Autodesk Fusion 360 part; units mm, degrees
sketch "Sketch1" plane through (0, 0, 0) normal (0, 0, 1) x (1, 0, 0)
  line L0 (0, 0) -> (7, 0)
  line L1 (7, 0) -> (7, 2)
  line L2 (7, 2) -> (0, 2)
  line L3 (0, 2) -> (0, 0)
  dimension "d1" = 7
  dimension "d2" = 2
extrude "Extrude1" add sketch "Sketch1" along normal blind 6
sketch "Sketch2" plane through (0, 2, 0) normal (0, 1, 0) x (-1, 0, 0)
  line L0 (-7, 0) -> (0, 0)
  line L1 (0, 0) -> (0, 6)
  line L2 (0, 6) -> (-7, 6)
  line L3 (-7, 6) -> (-7, 0)
  line L4 (-7, 3) -> (0, 3) construction
  line L5 (-3.5, 6) -> (-3.5, 0) construction
  circle A0 centre (-3.5, 3) radius 2.9
  circle A1 centre (-3.5, 3) radius 3.9
  line L6 (-5.2491, -0.4858) -> (-1.7509, -0.4858)
  line L7 (-5.2491, 6.4858) -> (-1.7509, 6.4858)
  dimension "d5" = 5.8
  dimension "d6" = 1
extrude "Extrude2" add sketch "Sketch2" along normal blind 5 contours L0 L1 L2 L3 A1 | L0 A1 L6 | L3 A1 | L1 A1 | L2 A1 L7
fillet "Fillet1" radius 1 4 edges at (0, 1, 6) (0, 1, 0) (7, 1, 0) (7, 1, 6)
fillet "Fillet2" radius 2 4 edges at (1.7509, 4.5, 6.4858) (5.2491, 4.5, 6.4858) (5.2491, 4.5, -0.4858) (1.7509, 4.5, -0.4858)
Part model, mm, in its own coordinate system. A direction names the side the tool comes from. Round coordinates to 2 decimals unless told otherwise and drop trailing zeros. Loops run counter-clockwise (first coordinate to the right, second up) from the corner with the lowest first, then second, coordinate; pieces in that order, holes last. Notation, with made-up numbers: (48, -22.75) - (97, -22.75) arc R8 ccw to (97, -14.75) - close; hole circle Ø2 at (0, 35). An arc over 180 degrees is marked (long way). Answer as a JSON object with one key per item and string values.
Item 1: Band-saw the part on A-A on y = 3.5. List the corners of the cut face in (x, z), plus the area to 3 significant figures.
Output:
{"outline": "(1.07, -0.05) arc R2 ccw to (2.32, -0.49) - (4.68, -0.49) arc R2 ccw to (5.93, -0.05) arc R3.9 ccw to (5.93, 6.05) arc R2 ccw to (4.68, 6.49) - (2.32, 6.49) arc R2 ccw to (1.07, 6.05) arc R3.9 ccw to start; hole circle Ø5.8 at (3.5, 3)", "area": "19.3 mm2"}
Item 2: Wall check: L1, parallel to Z at x = 3.5, y = 5.3; L2, parallel to Y at x = 4.5, z = 2.25; L3, parallel to X at y = 4.5, z = 3.75. Give the ranges that are in metal, low to high.
Output:
{"L1": "-0.49 to 0.1, 5.9 to 6.49", "L2": "0 to 2", "L3": "-0.33 to 0.7, 6.3 to 7.33"}
Item 3: Band-saw the part on C-C on z = 3. List the corners of the cut face in (x, y), plus the area to 3 significant figures.
Output:
{"outline": "(-0.4, 2) - (0, 2) - (0, 0) - (7, 0) - (7, 2) - (7.4, 2) - (7.4, 7) - (6.4, 7) - (6.4, 2) - (0.6, 2) - (0.6, 7) - (-0.4, 7) - close", "area": "24.0 mm2"}
Item 4: Band-saw the part on D-D on y = 1. List the corners of the cut face in (x, z).
Output:
{"outline": "(0, 1) arc R1 ccw to (1, 0) - (6, 0) arc R1 ccw to (7, 1) - (7, 5) arc R1 ccw to (6, 6) - (1, 6) arc R1 ccw to (0, 5) - close"}
Item 5: Pull direction X, two halves, no side cores. Call faces 1 (the face through (4, 2, 3)), 2 (the face through (4, 4, -0.486)), 3 (the face through (3.878, 4.465, 0.125)), 4 (the face through (6.715, 1.014, 0.301)): pulls with the +X half, pulls with the -X half, needs draft (parallel to the pull), parting line crosses it, or undercut.
Output:
{"face 1": "undercut", "face 2": "needs draft", "face 3": "undercut", "face 4": "pulls with the +X half"}
Item 6: Pin check, flat tips, straight feed: pin 1 (0.6 mm diameter, centred on y = 0.5, z = 3.5, fed in from -X); pin 2 (1.7 mm diameter, centred on x = 3, z = 4.5, fed in from +Y); pin 3 (1.6 mm diameter, centred on x = 2.5, y = 0.5, fed in from -Z). Stop position of each tip, or through.
Output:
{"pin 1": "x = 0", "pin 2": "y = 2", "pin 3": "z = 0"}
Item 7: Tool access for faces 5 (the face through (3, 1, 0)), 6 (the face through (0, 1, 3)), 7 (the face through (3, 1, 6)), 8 (the face through (7.4, 4.5, 3)): list every direction of +Z, -Z, +X, -X, +Y, -Y with a clear straight run to the whole face (end or side of a thin tool).
Output:
{"face 5": "-Z, +X, -X, -Y", "face 6": "+Z, -Z, -X, -Y", "face 7": "+Z, +X, -X, -Y", "face 8": "+X, +Y"}
Item 8: Band-saw the part on B-B on x = 3.5. List the corners of the cut face in (y, z).
Output:
{"outline": "(0, 0) - (2, 0) - (2, -0.49) - (7, -0.49) - (7, 0.1) - (2, 0.1) - (2, 5.9) - (7, 5.9) - (7, 6.49) - (2, 6.49) - (2, 6) - (0, 6) - close"}
